Geometry check sheet. Reference: the model listing, model coordinates, mm. Coordinates: 2 decimals unless noted, no trailing zeros. Order: outer loops, then holes, each group sorted by start corner. A loop starts at its lowest first (then second) coordinate and runs counter-clockwise, first axis right, second up. Notation, with made-up numbers: M 21,75.25 L 50,75.25 A31 ccw 50,99.25 Z; hole C 55,-14.5 d7. An arc over 180 degrees is marked long. One line per item, written item: value. Start each with the question number.
1) Thickness scan on L1, parallel to X at y = -127, z = 136; L2, parallel to X at y = -139.5, z = 142; L3, parallel to Y at x = 380.5, z = 364.5. Record the ranges inside material, lowest first. Write a range as from..to.
2) Go/stop test with flat-tipped pins: P1, Ø3, axis at y = -123.5, z = 404.5, coming from the +X side; P2, Ø1, axis at y = -86, z = 195.5, coming from the +X side; P3, Ø3, axis at y = 141.5, z = 365.5, coming from the -X side. Record where each tip stops, or that it passes through.
3) Sectioned sample at A-A, the plane z = 37. Enter the section's corners in (x, y).
4) Sectioned sample at B-B, the plane x = 315. Enter the section's corners in (y, z).
5) Sectioned sample at C-C, the plane y = 120.5. Enter the section's corners in (x, z).
```python
from build123d import *

# Parameters (mm, degrees)
ESQUISSE1_W        = 850
ESQUISSE1_H        = 150
BOSS_EXTRU_1_DEPTH = 500


with BuildPart() as part:
    # Esquisse1 → Boss.-Extru.1 (new body)
    with BuildSketch(Plane.XY):
        Polygon((404.882928221, 181.315844241), (254.882928221, 31.315844241), (404.882928221, 31.315844241), align=None)
        with Locations((829.882928221, 106.315844241)):
            Rectangle(ESQUISSE1_W, ESQUISSE1_H)
        Polygon((404.882928221, 31.315844241), (254.882928221, 31.315844241), (254.882928221, -73.684155759), (359.882928221, -178.684155759), (1149.882928221, -178.684155759), (1254.882928221, -73.684155759), (1254.882928221, 31.315844241), align=None)
    extrude(amount=BOSS_EXTRU_1_DEPTH)


solid = part.part
```
Final values:
1. L1: x = 308.2..1201.57
1. L2: x = 320.7..1189.07
1. L3: y = -178.68..156.93
2. P1: stops at x = 1206.57
2. P2: stops at x = 1243.07
2. P3: stops at x = 363.57
3. outline: M 254.88,-73.68 L 359.88,-178.68 L 1149.88,-178.68 L 1254.88,-73.68 L 1254.88,181.32 L 404.88,181.32 L 254.88,31.32 Z
4. outline: M -133.8,0 L 91.43,0 L 91.43,500 L -133.8,500 Z
5. outline: M 344.07,0 L 1254.88,0 L 1254.88,500 L 344.07,500 Z
